from build123d import *

# Parameters (mm, degrees)
SKETCH1_W                    = 21.59
SKETCH1_H                    = 41.91
SKETCH1_R                    = 4.124999878
BOSS_EXTRUDE1_DEPTH          = 3.175
EDGE_FLANGE2_STRIP_W         = 19.05
EDGE_FLANGE2_STRIP_H         = 3.175
EDGE_FLANGE2_STRIP_CUT_DEPTH = 21.59
EDGE_FLANGE2_DEPTH           = 21.59
EDGE_FLANGE2_FLAT_DEPTH      = 3.175
SKETCH12_R                   = 4.826
CUT_EXTRUDE1_DEPTH           = 79.776992708


# Sheet-metal steps are written as plain solids
with BuildPart() as part:
    # Sketch1 → Boss-Extrude1 (new body)
    with BuildSketch(Plane.XY):
        with Locations((10.795, 20.955)):
            Rectangle(SKETCH1_W, SKETCH1_H)
        with Locations(Location((10.795, 32.475227484, 0), (0, 0, 180))):
            Circle(SKETCH1_R, mode=Mode.SUBTRACT)
    extrude(amount=BOSS_EXTRUDE1_DEPTH)

    # Edge-Flange2 strip (across the edge) → Edge-Flange2 strip cut (cut)
    with BuildSketch(Plane(origin=(21.59, 0, 0), x_dir=(0, 1, 0), z_dir=(-1, 0, 0))):
        with Locations((-3.175, -1.5875)):
            Rectangle(EDGE_FLANGE2_STRIP_W, EDGE_FLANGE2_STRIP_H)
    extrude(amount=EDGE_FLANGE2_STRIP_CUT_DEPTH, mode=Mode.SUBTRACT)

    # Edge-Flange2 bend section (across the edge) → Edge-Flange2 (add)
    with BuildSketch(Plane(origin=(21.59, 0, 0), x_dir=(0, 1, 0), z_dir=(-1, 0, 0))):
        with BuildLine():
            Line((0, 3.175), (3.175, 3.175))
            ThreePointArc((3.175, 3.175), (4.10493597, 0.92993597), (6.35, 0))
            Line((6.35, 0), (6.35, -3.175))
            ThreePointArc((6.35, -3.175), (1.859871939, -1.315128061), (0, 3.175))
        make_face()
    extrude(amount=EDGE_FLANGE2_DEPTH)

    # Edge-Flange2 profile (on flange) → Edge-Flange2 flat (add)
    with BuildSketch(Plane(origin=(0, 0, 0), x_dir=(-1, 0, 0), z_dir=(0, -1, 0))):
        Polygon((0, 3.175), (0, 31.493260102), (27.326645128, 31.493260102), (46.376645128, 31.493260102), (46.376645128, 50.543260102), (27.326645128, 50.543260102), (0, 50.543260102), (-21.59, 50.543260102), (-21.59, 3.175), align=None)
    extrude(amount=-EDGE_FLANGE2_FLAT_DEPTH)

    # Sketch12 → Cut-Extrude1 (cut, through all)
    with BuildSketch(Plane(origin=(0, 3.175, 0), x_dir=(1, 0, 0), z_dir=(0, 1, 0))):
        with Locations(Location((-37.326625128, 41.493240102, 0), (0, 0, 270))):
            Circle(SKETCH12_R)
    extrude(amount=-CUT_EXTRUDE1_DEPTH, mode=Mode.SUBTRACT)


solid = part.part
Verification items for the finished model (mm, model axes). A direction names the side the tool comes from. Round coordinates to 2 decimals unless told otherwise and drop trailing zeros. Loops run counter-clockwise (first coordinate to the right, second up) from the corner with the lowest first, then second, coordinate; pieces in that order, holes last. Notation, with made-up numbers: (17, -31.75) - (42, -31.75) arc R13 ccw to (42, -6.75) - close; hole circle Ø1 at (83, -34.75). An arc over 180 degrees is marked (long way). Use a Markdown table: item, result. Add a question column.
1. Section check C-C, the plane x = -10. Record the boundary of the cut face in (y, z) (3 decimals).
2. Section check A-A, the plane z = -44. Record the boundary of the cut face in (x, y) (3 decimals).
3. Section check D-D, the plane y = 20. Record the boundary of the cut face in (x, z) (3 decimals).
4. Gauge pin test, flat ends, axial feed: pin 1 (1.6 mm diameter, centred on x = -30, y = 2, fed in from +Z); pin 2 (6.5 mm diameter, centred on x = 14.5, y = 18, fed in from -Z); pin 3 (10 mm diameter, centred on x = -22.5, z = -34.5, fed in from +Y) (3 decimals); pin 4 (7.5 mm diameter, centred on x = 10.8, y = 32.48, fed in from +Z). Record the tip position at first contact, or that the pin passes through.
5. Release check for a two-part mould opening along Z. For faces 4 (the face through (11, 24, 3.175)), 5 (the face through (-33.257, 1.61, -38.899)), 6 (the face through (21.59, 2, -12)), 7 (the face through (11, 24, 0)) record: released by +Z, released by -Z, zero draft, split by the parting line, or undercut.
6. Access from +Z, -Z, +X, -X, +Y, -Y to the whole of each face (thin tool, end or side, straight path). Record for faces 1 (the face through (0, 15, 1)), 2 (the face through (-4, 3.175, -32)), 3 (the face through (11, 41.91, 2)).
7. Section check B-B, the plane y = 33.5. Record the boundary of the cut face in (x, z) (3 decimals).
8. Thickness scan on probe 1 along Z at (x, y) = (6, 31.5) (3 decimals); probe 2 along X at (y, z) = (22, 1). Record the ranges inside material, lowest first. Write a range as [from, to].
Checks:
| question | item | result |
|---|---|---|
| 1 | outline | (0, -50.543) - (3.175, -50.543) - (3.175, -31.493) - (0, -31.493) - close |
| 2 | outline | (-46.377, 0) - (-41.451, 0) - (-41.451, 3.175) - (-46.377, 3.175) - close; (-33.203, 0) - (21.59, 0) - (21.59, 3.175) - (-33.203, 3.175) - close |
| 3 | outline | (0, 0) - (21.59, 0) - (21.59, 3.175) - (0, 3.175) - close |
| 4 | pin 1 | stops at z = -31.49 |
| 4 | pin 2 | stops at z = 0 |
| 4 | pin 3 | stops at y = 3.175 |
| 4 | pin 4 | passes through |
| 5 | face 4 | released by +Z |
| 5 | face 5 | undercut |
| 5 | face 6 | zero draft |
| 5 | face 7 | released by -Z |
| 6 | face 1 | +Z, -X, +Y, -Y |
| 6 | face 2 | -Z, +X, -X, +Y |
| 6 | face 3 | +Z, -Z, +X, -X, +Y |
| 7 | outline | (0, 0) - (6.799, 0) - (6.799, 3.175) - (0, 3.175) - close; (14.791, 0) - (21.59, 0) - (21.59, 3.175) - (14.791, 3.175) - close |
| 8 | probe 1 | z = [0, 3.175] |
| 8 | probe 2 | x = [0, 21.59] |
